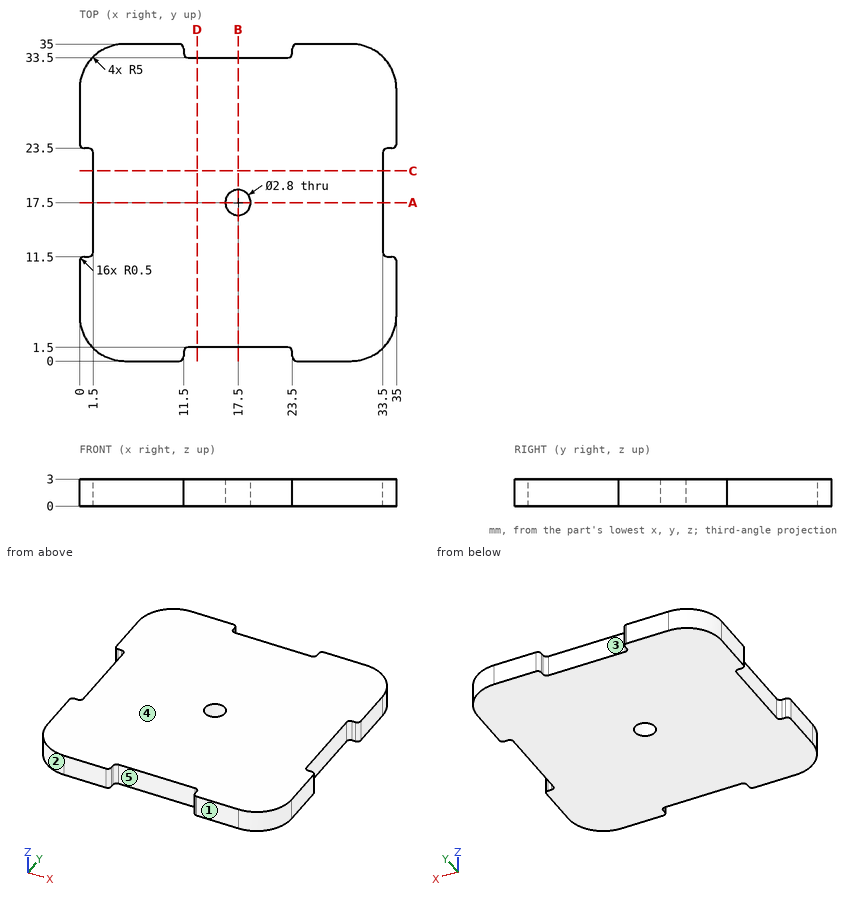
Input: dimensioned drawing with shaded views. Units: mm. Origin: part minimum x, y, z. A direction names the side the tool comes from. Coordinates: 2 decimals unless noted, no trailing zeros. Write each loop counter-clockwise with the first axis right and the second up, starting at its lowest first coordinate (ties: lowest second). Pieces come first, ordered by that corner, then holes. Notation, with made-up numbers: M -26,3 L -7,3 A3 cw -7,7 Z; hole C -38,72.25 d3. An arc over 180 degrees is marked long. Use one line per item in the form item = value.
Q1. First-contact query: pin 1 (0.6 mm diameter, centred on y = 0.5, z = 2, fed in from +X); pin 2 (0.6 mm diameter, centred on x = 0.5, z = 1, fed in from +Y); pin 3 (0.9 mm diameter, centred on y = 18, z = 1.5, fed in from +X). Flat tips, straight axial feed; report the tip coordinate or a pass-through.
Answer below:
pin_1 = 32.71
pin_2 = 32.71
pin_3 = 33.5
Q2. Draft query along X for the marked faces 1, 2 and 3. Return one class per face: released by +X, released by -X, zero draft, split by the parting line, or undercut.
Answer below:
face_1 = zero draft
face_2 = released by -X
face_3 = undercut
Q3. Set-up query: the marked faces 4 and 5. Return all of +Z, -Z, +X, -X, +Y, -Y with unobstructed straight access to the full face (end or side cutting, diameter ignored); none if empty.
Answer below:
face_4 = +Z, +X, -X, +Y, -Y
face_5 = +Z, -Z, -Y
Q4. Section A-A (y = 17.5). Return loops of the section in (x, z), plus the area to 3 significant figures.
Answer below:
outline = M 1.5,0 L 16.1,0 L 16.1,3 L 1.5,3 Z; M 18.9,0 L 33.5,0 L 33.5,3 L 18.9,3 Z
area = 87.6 mm²
Q5. Material intervals for probe 1 along Y at (x, z) = (17.5, 1.6); probe 2 along X at (y, z) = (12, 0.6), sorted ascending. Write a range as from..to.
Answer below:
probe_1 = 1.5..16.1, 18.9..33.5
probe_2 = 1.5..33.5
Q6. Section C-C (y = 21). Return loops of the section in (x, z), plus the area to 3 significant figures.
Answer below:
outline = M 1.5,0 L 33.5,0 L 33.5,3 L 1.5,3 Z
area = 96.0 mm²
